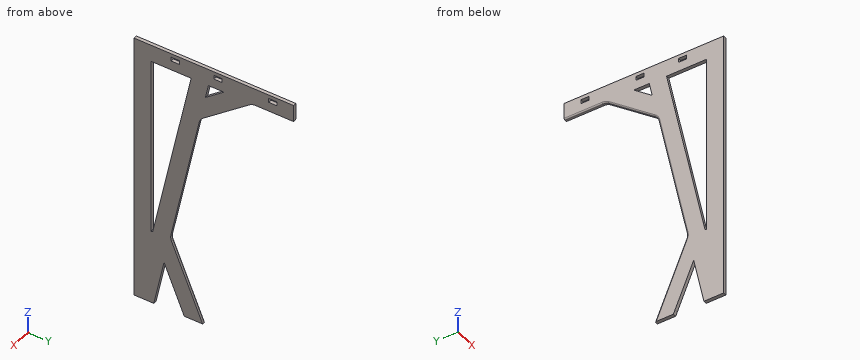
```python
from build123d import *

# Parameters (mm, degrees)
F1_DEPTH = 2.1082
F2_R     = 0.762


# Not quite as in the source:
# - a feature names something its author has since deleted; it is built from what else it names


with BuildPart() as f1:
    # F0 (on Right) → F1 (new body)
    with BuildSketch(Plane.YZ):
        with BuildLine():
            Line((0, 169.3418), (0, 0))
            Line((0, 0), (12.335197777, 0))
            Line((12.335197777, 0), (18.8042013144, 29.896105485))
            Line((18.8042013144, 29.896105485), (30.5493542935, 2.3257501254))
            Line((30.5493542935, 2.3257501254), (31.5401391658, 0))
            Line((31.5401391658, 0), (31.5707651968, 0))
            Line((31.5707651968, 0), (40.8442968098, 0))
            Line((40.8442968098, 0), (20.5594925834, 47.616175108))
            Line((20.5594925834, 47.616175108), (39.5771112022, 135.5049402038))
            Line((39.5771112022, 135.5049402038), (73.5248959406, 160.7899383022))
            Line((73.5248959406, 160.7899383022), (100.203, 160.7899383022))
            Line((100.203, 160.7899383022), (100.203, 162.0091375))
            Line((100.203, 162.0091375), (82.1398573303, 162.0091375))
            ThreePointArc((82.1398573303, 162.0091375), (80.3438061061, 162.7530862758), (79.5998573303, 164.5491375))
            Line((79.5998573303, 164.5491375), (79.5998573303, 169.3418))
            Line((79.5998573303, 169.3418), (70.6874244764, 169.3418))
            Line((70.6874244764, 169.3418), (70.6874244764, 165.8480664454))
            Line((70.6874244764, 165.8480664454), (70.6874244764, 164.5491375))
            ThreePointArc((70.6874244764, 164.5491375), (70.0510915867, 162.8675752701), (68.4609272063, 162.0285589874))
            ThreePointArc((68.4609272063, 162.0285589874), (68.3044763435, 162.0139975214), (68.1474244764, 162.0091375))
            Line((68.1474244764, 162.0091375), (18.2118, 162.0091375))
            ThreePointArc((18.2118, 162.0091375), (16.4157487758, 162.7530862758), (15.6718, 164.5491375))
            Line((15.6718, 164.5491375), (15.6718, 169.3418))
            Line((15.6718, 169.3418), (0, 169.3418))
        make_face()
        Polygon((21.4843682503, 35.8535070154), (23.4753466245, 31.1799211209), (21.1385536773, 30.1844319338), (19.147575303, 34.8580178283), align=None, mode=Mode.SUBTRACT)
        Polygon((25.8665425285, 25.5668719827), (27.8575209028, 20.8932860882), (25.5207279555, 19.8977969011), (23.5297495813, 24.5713827956), align=None, mode=Mode.SUBTRACT)
        with BuildLine():
            Line((12.3986134924, 50.3752630702), (11.6175919588, 46.7658196656))
            Line((11.6175919588, 46.7658196656), (10.5918, 46.7658196656))
            Line((10.5918, 46.7658196656), (10.5918, 158.7579375))
            Line((10.5918, 158.7579375), (35.8507619547, 158.7579375))
            Line((35.8507619547, 158.7579375), (31.8897708968, 140.4524587956))
            Line((31.8897708968, 140.4524587956), (31.1087493632, 136.8430153909))
            Line((31.1087493632, 136.8430153909), (35.5475592049, 135.882533211))
            ThreePointArc((35.5475592049, 135.882533211), (37.1456481821, 134.7755682604), (37.4929253116, 132.8628062845))
            Line((37.4929253116, 132.8628062845), (29.5595533377, 96.1992113407))
            ThreePointArc((29.5595533377, 96.1992113407), (28.452588387, 94.6011223635), (26.5398264112, 94.2538452339))
            Line((26.5398264112, 94.2538452339), (22.1010165695, 95.2143274138))
            Line((22.1010165695, 95.2143274138), (21.7536814278, 93.6091392306))
            Line((21.7536814278, 93.6091392306), (21.4063462861, 92.0039510473))
            Line((21.4063462861, 92.0039510473), (25.8451561277, 91.0434688674))
            ThreePointArc((25.8451561277, 91.0434688674), (27.4432451049, 89.9365039168), (27.7905222345, 88.0237419409))
            Line((27.7905222345, 88.0237419409), (19.8571502605, 51.3601469971))
            ThreePointArc((19.8571502605, 51.3601469971), (18.7501853099, 49.7620580199), (16.837423334, 49.4147808903))
            Line((16.837423334, 49.4147808903), (12.3986134924, 50.3752630702))
        make_face(mode=Mode.SUBTRACT)
        Polygon((47.0613097153, 149.2568137468), (48.5785484084, 147.2197602993), (44.5044415132, 144.1852829132), (42.9872028202, 146.2223363607), align=None, mode=Mode.SUBTRACT)
        Polygon((44.8088104432, 150.074821282), (46.6876875952, 158.7579375), (56.4668125154, 158.7579375), align=None, mode=Mode.SUBTRACT)
        Polygon((63.2751536106, 161.3332132886), (64.7923923036, 159.296159841), (60.7182854085, 156.2616824549), (59.2010467154, 158.2987359025), align=None, mode=Mode.SUBTRACT)
        with BuildLine():
            Line((20.5594925834, 47.616175108), (40.8442968098, 0))
            Line((40.8442968098, 0), (43.053, 0))
            Line((43.053, 0), (23.4736756901, 45.9601445708))
            ThreePointArc((23.4736756901, 45.9601445708), (22.9941781878, 47.847708452), (23.1092917667, 49.7918185633))
            Line((23.1092917667, 49.7918185633), (40.8984089502, 132.0031391675))
            ThreePointArc((40.8984089502, 132.0031391675), (41.765080018, 134.0967787378), (43.3116785091, 135.7528217618))
            Line((43.3116785091, 135.7528217618), (72.5103326221, 157.500571119))
            ThreePointArc((72.5103326221, 157.500571119), (74.3053957564, 158.4354047741), (76.3034293547, 158.7579375))
            Line((76.3034293547, 158.7579375), (100.203, 158.7579375))
            Line((100.203, 158.7579375), (100.203, 160.7899383022))
            Line((100.203, 160.7899383022), (73.5248959406, 160.7899383022))
            Line((73.5248959406, 160.7899383022), (39.5771112022, 135.5049402038))
            Line((39.5771112022, 135.5049402038), (20.5594925834, 47.616175108))
        make_face()
        Polygon((68.1474244764, 169.3418), (18.2118, 169.3418), (18.2118, 164.5491375), (23.2918, 164.5491375), (23.2918, 167.0891375), (28.3718, 167.0891375), (28.3718, 164.5491375), (50.0948093832, 164.5491375), (50.0948093832, 167.0891375), (55.1748093832, 167.0891375), (55.1748093832, 164.5491375), (68.1474244764, 164.5491375), (68.1474244764, 165.0060867035), align=None)
        with BuildLine():
            Line((18.2118, 169.3418), (15.6718, 169.3418))
            Line((15.6718, 169.3418), (15.6718, 164.5491375))
            ThreePointArc((15.6718, 164.5491375), (16.4157487758, 162.7530862758), (18.2118, 162.0091375))
            Line((18.2118, 162.0091375), (68.1474244764, 162.0091375))
            ThreePointArc((68.1474244764, 162.0091375), (68.3044763435, 162.0139975214), (68.4609272063, 162.0285589874))
            Line((68.4609272063, 162.0285589874), (69.6856973646, 162.9407926238))
            Line((69.6856973646, 162.9407926238), (68.1474244764, 165.0060867035))
            Line((68.1474244764, 165.0060867035), (68.1474244764, 164.5491375))
            Line((68.1474244764, 164.5491375), (55.1748093832, 164.5491375))
            Line((55.1748093832, 164.5491375), (50.0948093832, 164.5491375))
            Line((50.0948093832, 164.5491375), (28.3718, 164.5491375))
            Line((28.3718, 164.5491375), (23.2918, 164.5491375))
            Line((23.2918, 164.5491375), (18.2118, 164.5491375))
            Line((18.2118, 164.5491375), (18.2118, 169.3418))
        make_face()
        Polygon((20.8691658762, 89.5214045307), (12.9357939022, 52.8578095868), (17.3746037439, 51.8973274069), (18.6675621562, 57.872655888), (16.1850156395, 58.4098362979), (17.2593764593, 63.3749293312), (19.7419229759, 62.8377489213), (22.9432277355, 77.6323837102), (20.4606812189, 78.16956412), (21.5350420386, 83.1346571533), (24.0175885553, 82.5974767434), (25.3079757178, 88.5609223508), align=None)
        Polygon((35.010378795, 133.3999866944), (30.5715689534, 134.3604688743), (22.6381969794, 97.6968739305), (27.077006821, 96.7363917505), (28.3673939836, 102.6998373579), (25.884847467, 103.2370177677), (26.9592082867, 108.202110801), (29.4417548033, 107.6649303911), (32.643059563, 122.45956518), (30.1605130463, 122.9967455899), (31.2348738661, 127.9618386231), (33.7174203827, 127.4246582133), align=None)
        with BuildLine():
            Line((12.9357939022, 52.8578095868), (12.3986134924, 50.3752630702))
            Line((12.3986134924, 50.3752630702), (16.837423334, 49.4147808903))
            ThreePointArc((16.837423334, 49.4147808903), (18.7501853099, 49.7620580199), (19.8571502605, 51.3601469971))
            Line((19.8571502605, 51.3601469971), (27.7905222345, 88.0237419409))
            ThreePointArc((27.7905222345, 88.0237419409), (27.4432451049, 89.9365039168), (25.8451561277, 91.0434688674))
            Line((25.8451561277, 91.0434688674), (21.4063462861, 92.0039510473))
            Line((21.4063462861, 92.0039510473), (20.8691658762, 89.5214045307))
            Line((20.8691658762, 89.5214045307), (25.3079757178, 88.5609223508))
            Line((25.3079757178, 88.5609223508), (24.0175885553, 82.5974767434))
            Line((24.0175885553, 82.5974767434), (22.9432277355, 77.6323837102))
            Line((22.9432277355, 77.6323837102), (19.7419229759, 62.8377489213))
            Line((19.7419229759, 62.8377489213), (18.6675621562, 57.872655888))
            Line((18.6675621562, 57.872655888), (17.3746037439, 51.8973274069))
            Line((17.3746037439, 51.8973274069), (12.9357939022, 52.8578095868))
        make_face()
        with BuildLine():
            Line((35.5475592049, 135.882533211), (31.1087493632, 136.8430153909))
            Line((31.1087493632, 136.8430153909), (30.5715689534, 134.3604688743))
            Line((30.5715689534, 134.3604688743), (35.010378795, 133.3999866944))
            Line((35.010378795, 133.3999866944), (33.7174203827, 127.4246582133))
            Line((33.7174203827, 127.4246582133), (32.643059563, 122.45956518))
            Line((32.643059563, 122.45956518), (29.4417548033, 107.6649303911))
            Line((29.4417548033, 107.6649303911), (28.3673939836, 102.6998373579))
            Line((28.3673939836, 102.6998373579), (27.077006821, 96.7363917505))
            Line((27.077006821, 96.7363917505), (22.6381969794, 97.6968739305))
            Line((22.6381969794, 97.6968739305), (22.1010165695, 95.2143274138))
            Line((22.1010165695, 95.2143274138), (26.5398264112, 94.2538452339))
            ThreePointArc((26.5398264112, 94.2538452339), (28.452588387, 94.6011223635), (29.5595533377, 96.1992113407))
            Line((29.5595533377, 96.1992113407), (37.4929253116, 132.8628062845))
            ThreePointArc((37.4929253116, 132.8628062845), (37.1456481821, 134.7755682604), (35.5475592049, 135.882533211))
        make_face()
        Polygon((100.203, 169.3418), (82.1398573303, 169.3418), (82.1398573303, 164.5491375), (84.5702663064, 164.5491375), (84.5702663064, 167.0891375), (89.6502663064, 167.0891375), (89.6502663064, 164.5491375), (100.203, 164.5491375), align=None)
        with BuildLine():
            Line((82.1398573303, 169.3418), (79.5998573303, 169.3418))
            Line((79.5998573303, 169.3418), (79.5998573303, 164.5491375))
            ThreePointArc((79.5998573303, 164.5491375), (80.3438061061, 162.7530862758), (82.1398573303, 162.0091375))
            Line((82.1398573303, 162.0091375), (100.203, 162.0091375))
            Line((100.203, 162.0091375), (100.203, 164.5491375))
            Line((100.203, 164.5491375), (89.6502663064, 164.5491375))
            Line((89.6502663064, 164.5491375), (84.5702663064, 164.5491375))
            Line((84.5702663064, 164.5491375), (82.1398573303, 164.5491375))
            Line((82.1398573303, 164.5491375), (82.1398573303, 169.3418))
        make_face()
        with BuildLine():
            Line((70.6874244764, 169.3418), (68.1474244764, 169.3418))
            Line((68.1474244764, 169.3418), (68.1474244764, 165.0060867035))
            Line((68.1474244764, 165.0060867035), (69.6856973646, 162.9407926238))
            Line((69.6856973646, 162.9407926238), (68.4609272063, 162.0285589874))
            ThreePointArc((68.4609272063, 162.0285589874), (70.0510915867, 162.8675752701), (70.6874244764, 164.5491375))
            Line((70.6874244764, 164.5491375), (70.6874244764, 165.8480664454))
            Line((70.6874244764, 165.8480664454), (70.6874244764, 169.3418))
        make_face()
        Polygon((21.1385536773, 30.1844319338), (23.4753466245, 31.1799211209), (21.4843682503, 35.8535070154), (19.147575303, 34.8580178283), align=None)
        Polygon((25.5207279555, 19.8977969011), (27.8575209028, 20.8932860882), (25.8665425285, 25.5668719827), (23.5297495813, 24.5713827956), align=None)
        Polygon((44.5044415132, 144.1852829132), (48.5785484084, 147.2197602993), (47.0613097153, 149.2568137468), (42.9872028202, 146.2223363607), align=None)
        Polygon((60.7182854085, 156.2616824549), (64.7923923036, 159.296159841), (63.2751536106, 161.3332132886), (59.2010467154, 158.2987359025), align=None)
        Polygon((16.1850156395, 58.4098362979), (18.6675621562, 57.872655888), (19.7419229759, 62.8377489213), (17.2593764593, 63.3749293312), align=None)
        Polygon((22.9432277355, 77.6323837102), (24.0175885553, 82.5974767434), (21.5350420386, 83.1346571533), (20.4606812189, 78.16956412), align=None)
        Polygon((32.643059563, 122.45956518), (33.7174203827, 127.4246582133), (31.2348738661, 127.9618386231), (30.1605130463, 122.9967455899), align=None)
        Polygon((25.884847467, 103.2370177677), (28.3673939836, 102.6998373579), (29.4417548033, 107.6649303911), (26.9592082867, 108.202110801), align=None)
    extrude(amount=F1_DEPTH)

    # F2
    f2_edges = [f1.edges().sort_by_distance(p)[0] for p in [
        (0, 32.00385, 90.897479),
        (0, 33.263338, 22.980072),
        (0, 22.994178, 47.847708),
        (0, 41.76508, 134.096779),
        (0, 57.911006, 146.626696),
        (0, 74.305396, 158.435405),
        (0, 88.253215, 158.757937),
    ]]
    fillet(f2_edges, radius=F2_R)


solid = f1.part
```
Can you work these out from the model? Positions are in its coordinate system, mm. Give positions to 0.01 mm unless a question says otherwise; leave off trailing zeros. Write each loop counter-clockwise with the first axis right and the second up, starting at its lowest first coordinate (ties: lowest second). Pieces come first, ordered by that corner, then holes. Notation, with made-up numbers: (13, 46.25) - (36, 46.25) arc R21 ccw to (36, 55.25) - close; hole circle Ø3 at (21, 66). An arc over 180 degrees is marked (long way). Write item = value, one per line. Start each with the question number.
1. For pin 1 (1.1 mm diameter, centred on x = 1.5, z = 165.5, fed in from -Y); pin 2 (0.6 mm diameter, centred on x = 1, y = 52, fed in from -Z); pin 3 (1.1 mm diameter, centred on x = 1, z = 76.5, fed in from +Y); pin 4 (1.1 mm diameter, centred on x = 1.5, y = 51.5, fed in from -Z), each with a flat end and sliding along its axis, tell me the tip position at first contact or that it passes through.
2. Imagine slicing it at B-B (x = 1.3). Count the separate pieces of the cut face and the enclosed holes in it, and give its area (3 significant figures).
3. Please list where these lines run through material, in increasing order: line 1 (Y direction, x = 1.15, z = 150.5); line 2 (Z direction, x = 0.85, y = 11); line 3 (Z direction, x = 0.9, y = 77.5).
4. Imagine slicing it at A-A (y = 82). Please give me the cut outline in (x, z).
Worked answers:
q1.pin_1 = 0
q1.pin_2 = 142
q1.pin_3 = 29.01
q1.pin_4 = 141.44
q2.separate_pieces = 1
q2.enclosed_holes = 5
q2.area = 4,980 mm2
q3.line_1 = 0 to 10.59, 34.06 to 44.9, 45.38 to 63.11
q3.line_2 = 0 to 46.77, 158.76 to 169.34
q3.line_3 = 158.76 to 169.34
q4.outline = (0, 159.52) arc R0.76 ccw to (0.76, 158.76) - (2.11, 158.76) - (2.11, 169.34) - (0, 169.34) - close
